from build123d import *

# Parameters (mm, degrees)
SKETCH1_W                 = 114
SKETCH1_H                 = 31
BOSS_EXTRUDE1_DEPTH       = 10
SKETCH2_W                 = 114
SKETCH2_H                 = 6
CUT_EXTRUDE1_DEPTH        = 5
M2X0_4_TAPPED_HOLE1_D     = 1.6
M2X0_4_TAPPED_HOLE1_DEPTH = 7
M2X0_4_TAPPED_HOLE1_TIP   = 0.480688495
M2X0_4_TAPPED_HOLE3_D     = 1.6
M2X0_4_TAPPED_HOLE3_DEPTH = 7
M2X0_4_TAPPED_HOLE3_TIP   = 0.480688495
M2X0_4_TAPPED_HOLE2_D     = 1.6
M2X0_4_TAPPED_HOLE2_DEPTH = 7
M2X0_4_TAPPED_HOLE2_TIP   = 0.480688495


with BuildPart() as part:
    # Sketch1 → Boss-Extrude1 (new body)
    with BuildSketch(Plane.XY):
        with Locations((57, 15.5)):
            Rectangle(SKETCH1_W, SKETCH1_H)
    extrude(amount=BOSS_EXTRUDE1_DEPTH)

    # Sketch2 → Cut-Extrude1 (cut)
    with BuildSketch(Plane.XY.offset(10)):
        with Locations((57, 28)):
            Rectangle(SKETCH2_W, SKETCH2_H)
    extrude(amount=-CUT_EXTRUDE1_DEPTH, mode=Mode.SUBTRACT)

    # M2x0.4 Tapped Hole1
    with Locations(Plane(origin=(0, 14, 5), x_dir=(0, 0, -1), z_dir=(-1, 0, 0))):
        with Locations((0, 0), (0, 8)):
            Hole(M2X0_4_TAPPED_HOLE1_D / 2, depth=M2X0_4_TAPPED_HOLE1_DEPTH)
            with Locations((0, 0, -(M2X0_4_TAPPED_HOLE1_DEPTH + M2X0_4_TAPPED_HOLE1_TIP / 2))):  # 118° drill point
                Cone(0, M2X0_4_TAPPED_HOLE1_D / 2, M2X0_4_TAPPED_HOLE1_TIP, mode=Mode.SUBTRACT)

    # M2x0.4 Tapped Hole3
    with Locations(Plane(origin=(114, 14, 5), x_dir=(0, 0, 1), z_dir=(1, 0, 0))):
        with Locations((0, 0), (0, 8)):
            Hole(M2X0_4_TAPPED_HOLE3_D / 2, depth=M2X0_4_TAPPED_HOLE3_DEPTH)
            with Locations((0, 0, -(M2X0_4_TAPPED_HOLE3_DEPTH + M2X0_4_TAPPED_HOLE3_TIP / 2))):  # 118° drill point
                Cone(0, M2X0_4_TAPPED_HOLE3_D / 2, M2X0_4_TAPPED_HOLE3_TIP, mode=Mode.SUBTRACT)

    # M2x0.4 Tapped Hole2
    with Locations(Plane(origin=(0, 0, 0), x_dir=(-1, 0, 0), z_dir=(0, -1, 0))):
        with Locations((-102, -5), (-12, -5), (-57, -5), (-79, -5), (-35, -5)):
            Hole(M2X0_4_TAPPED_HOLE2_D / 2, depth=M2X0_4_TAPPED_HOLE2_DEPTH)
            with Locations((0, 0, -(M2X0_4_TAPPED_HOLE2_DEPTH + M2X0_4_TAPPED_HOLE2_TIP / 2))):  # 118° drill point
                Cone(0, M2X0_4_TAPPED_HOLE2_D / 2, M2X0_4_TAPPED_HOLE2_TIP, mode=Mode.SUBTRACT)


solid = part.part
Can you work these out from the model? Positions are in its coordinate system, mm. A direction names the side the tool comes from. Give positions to 0.01 mm unless a question says otherwise; leave off trailing zeros. Write each loop counter-clockwise with the first axis right and the second up, starting at its lowest first coordinate (ties: lowest second). Pieces come first, ordered by that corner, then holes. Notation, with made-up numbers: (49, 3) -> (70, 3) arc R13 ccw to (70, 28) -> close; hole circle Ø11 at (84.5, 22). An arc over 180 degrees is marked (long way). Answer as a JSON object with one key per item and string values. Group by question number.
Item 1: Suppose I cut it at C-C (z = 7). Please give me the cut outline in (x, y), plus the area to 3 significant figures.
Item 2: I'm going to push flat-ended pins straight in: P1, Ø1.5, axis at x = 82.5, z = 6.5, coming from the +Y side; P2, Ø1.4, axis at y = 6, z = 5, coming from the -X side; P3, Ø6.5, axis at x = 52.5, y = 28.5, coming from the +Z side. Where does each tip first touch, or does it pass through?
Item 3: Please list where these lines run through material, in increasing order: line 1 (X direction, y = 2.5, z = 5); line 2 (Z direction, x = 109.75, y = 14); line 3 (Y direction, x = 89, z = 5.25). Write a range as [from, to].
Item 4: Suppose I cut it at B-B (y = 26). Please give me the cut outline in (x, z).
Item 5: For faces 1 (the face through (56, 13, 10)), 2 (the face through (56, 25, 8)), which set-ups out of +Z, -Z, +X, -X, +Y, -Y let a thin tool reach every point of the face, with its end or its side?
Item 6: Suppose I cut it at A-A (x = 55). Please give me the cut outline in (y, z).
Findings:
{
 "1": {"outline": "(0, 0) -> (114, 0) -> (114, 25) -> (0, 25) -> close", "area": "2,850 mm²"},
 "2": {"P1": "stops at y = 25", "P2": "stops at x = 7.06", "P3": "stops at z = 5"},
 "3": {"line 1": "x = [0, 11.2], [12.8, 34.2], [35.8, 56.2], [57.8, 78.2], [79.8, 101.2], [102.8, 114]", "line 2": "z = [0, 4.2], [5.8, 10]", "line 3": "y = [0, 25]"},
 "4": {"outline": "(0, 0) -> (114, 0) -> (114, 5) -> (0, 5) -> close"},
 "5": {"face 1": "+Z, +X, -X, +Y, -Y", "face 2": "+Z, +X, -X, +Y"},
 "6": {"outline": "(0, 0) -> (31, 0) -> (31, 5) -> (25, 5) -> (25, 10) -> (0, 10) -> close"}
}
